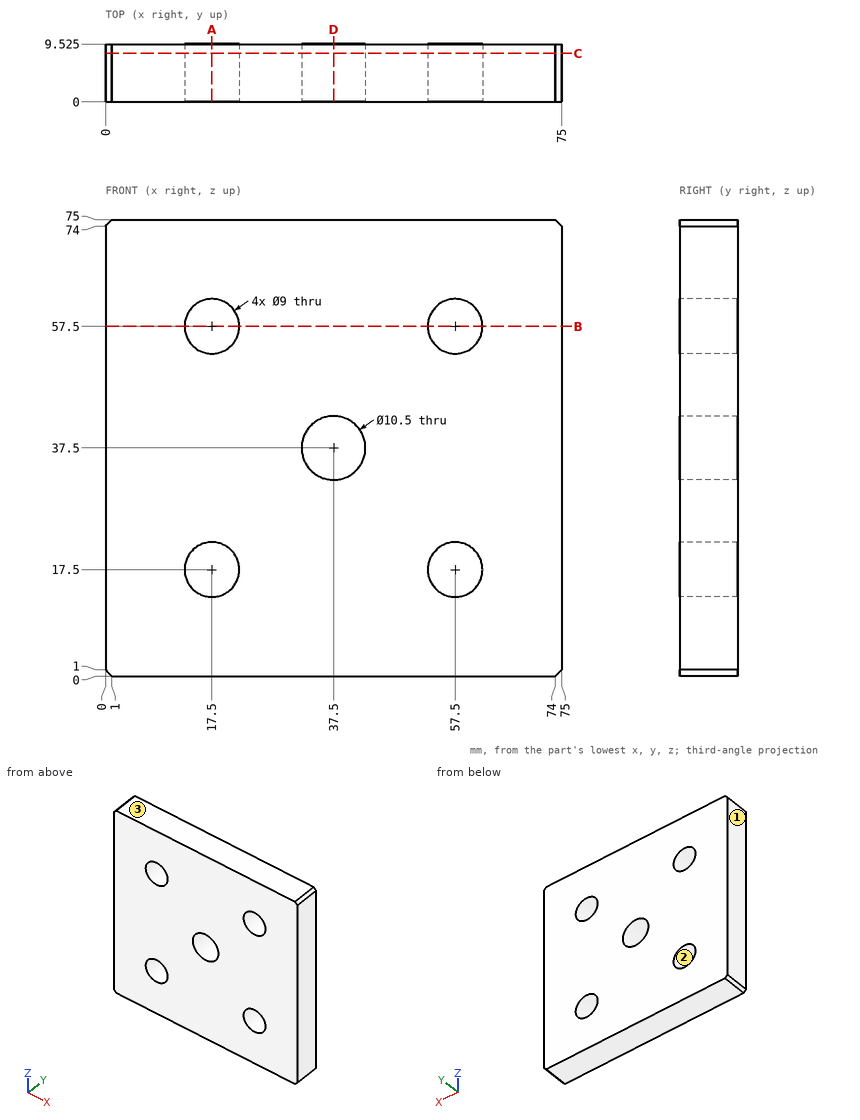
For this review, use the dimensioned drawing (mm, ordinates from the lowest corner) and the shaded views. Give positions to 0.01 mm unless a question says otherwise; leave off trailing zeros. Order: outer loops, then holes, each group sorted by start corner. A loop starts at its lowest first (then second) coordinate and runs counter-clockwise, first axis right, second up. Notation, with made-up numbers: M 30.25,-0.75 L 89.25,-0.75 A18 cw 89.25,24.25 Z; hole C -32,39.25 d10. An arc over 180 degrees is marked long. Use one line per item in the form item = value. Start each with the question number.
Item 1: We need section A-A on x = 17.5. Give the boundary of the cut face in (y, z) (3 decimals), plus the area to 3 significant figures.
Item 2: We need section C-C on y = 8. Give the boundary of the cut face in (x, z), plus the area to 3 significant figures.
Item 3: Insertion check: pin 1 Ø7 at (x, z) = (57.5, 17.5) entering from -Y; pin 2 Ø5 at (y, z) = (5, 48.5) entering from -X. Each pin has a flat end and moves straight along its axis. Give the tip position at first contact, or say it passes through.
Item 4: To check wall thickness, follow line 1 along X through (y, z) = (2, 17.5); line 2 along X through (y, z) = (2.75, 37.5). State the ranges of each line that lie inside material, in increasing order. Write a range as from..to.
Item 5: The part is to be moulded in two halves that separate along X. For the marked faces 1, 2 and 3, say which applies: pulls with the +X half, pulls with the -X half, needs draft (parallel to the pull), parting line crosses it, or undercut.
Item 6: We need section B-B on z = 57.5. Give the boundary of the cut face in (x, y) (3 decimals).
Item 7: We need section D-D on x = 37.5. Give the boundary of the cut face in (y, z) (3 decimals).
Completed:
q1.outline = M 0,0 L 9.525,0 L 9.525,13 L 0,13 Z; M 0,22 L 9.525,22 L 9.525,53 L 0,53 Z; M 0,62 L 9.525,62 L 9.525,75 L 0,75 Z
q1.area = 543 mm²
q2.outline = M 0,1 L 1,0 L 74,0 L 75,1 L 75,74 L 74,75 L 1,75 L 0,74 Z; hole C 17.5,17.5 d9; hole C 17.5,57.5 d9; hole C 37.5,37.5 d10.5; hole C 57.5,17.5 d9; hole C 57.5,57.5 d9
q2.area = 5,280 mm²
q3.pin_1 = through
q3.pin_2 = 0
q4.line_1 = 0..13, 22..53, 62..75
q4.line_2 = 0..32.25, 42.75..75
q5.face_1 = pulls with the -X half
q5.face_2 = undercut
q5.face_3 = needs draft
q6.outline = M 0,0 L 13,0 L 13,9.525 L 0,9.525 Z; M 22,0 L 53,0 L 53,9.525 L 22,9.525 Z; M 62,0 L 75,0 L 75,9.525 L 62,9.525 Z
q7.outline = M 0,0 L 9.525,0 L 9.525,32.25 L 0,32.25 Z; M 0,42.75 L 9.525,42.75 L 9.525,75 L 0,75 Z
